The figure shows three views and two pictorial views of one solid part (mm, origin at its lowest corner). Answer the questions. A direction names the side the tool comes from. Give positions to 0.01 mm unless a question says otherwise; leave off trailing zeros. Loops run counter-clockwise (first coordinate to the right, second up) from the corner with the lowest first, then second, coordinate; pieces in that order, holes last. Notation, with made-up numbers: M 41,-40 L 63,-40 A36 ccw 63,-4 Z; hole C 46,32 d10. An arc over 180 degrees is marked long. Write item = value, one per line. Start each with the question number.
1. Section A-A on y = 20 is taken. Determine the outline of the cut face in (x, z), plus the area to 3 significant figures.
2. Section C-C on x = 194 is taken. Determine the outline of the cut face in (y, z), plus the area to 3 significant figures.
3. For the marked faces 1, 2 and 3, determine the directions among +Z, -Z, +X, -X, +Y, -Y from which every point of the face is accessible in a straight line to the end or side of a thin tool.
4. Section D-D on z = 36 is taken. Determine the outline of the cut face in (x, y).
5. Consider L1, parallel to X at y = 10, z = 30; L2, parallel to X at y = 31.5, z = 19.5; L3, parallel to Z at x = 168, y = 20. Determine where each line is inside the solid, lowest interval first. Write a range as [from, to].
6. Flat-ended cylindrical pins translate along their axes: pin 1 Ø10 at (y, z) = (4.5, 23.5) entering from +X; pin 2 Ø1.5 at (x, z) = (146.5, 31.5) entering from -Y; pin 3 Ø1 at (y, z) = (30, 31) entering from -X; pin 4 Ø4 at (x, y) = (245.5, 36) entering from -Z. Find the tip coordinate at first contact, or state that the pin passes through.
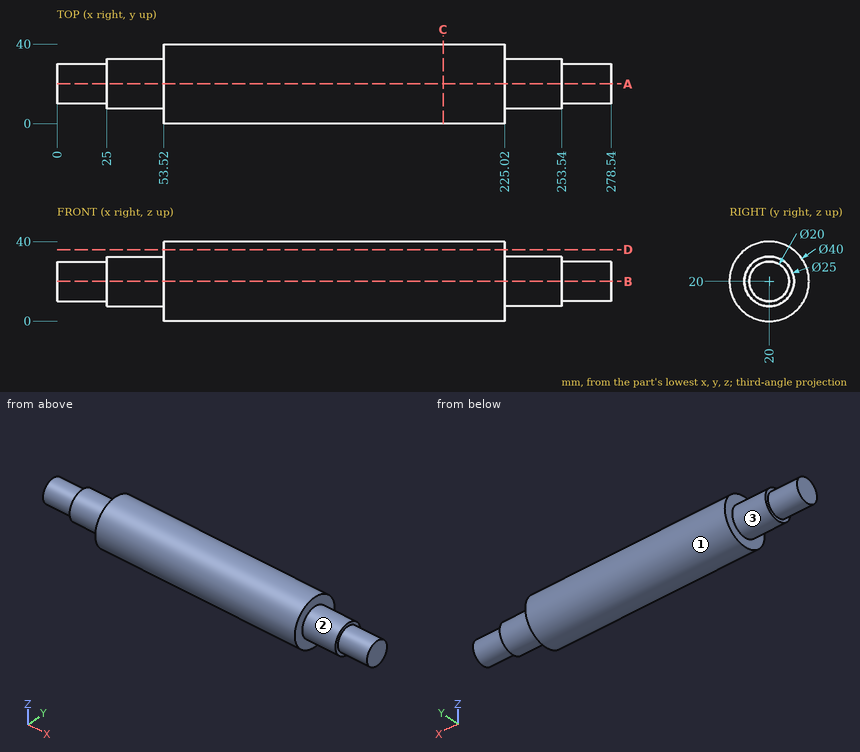
Verdict:
q1.outline = M 0,10 L 25,10 L 25,7.5 L 53.52,7.5 L 53.52,0 L 225.02,0 L 225.02,7.5 L 253.54,7.5 L 253.54,10 L 278.54,10 L 278.54,30 L 253.54,30 L 253.54,32.5 L 225.02,32.5 L 225.02,40 L 53.52,40 L 53.52,32.5 L 25,32.5 L 25,30 L 0,30 Z
q1.area = 9,290 mm2
q2.outline = C 20,20 d40
q2.area = 1,260 mm2
q3.face_1 = +X, -X
q3.face_2 = +X
q3.face_3 = -X
q4.outline = M 53.52,8 L 225.02,8 L 225.02,32 L 53.52,32 Z
q5.L1 = [53.52, 225.02]
q5.L2 = [25, 253.54]
q5.L3 = [0, 40]
q6.pin_1 = 253.54
q6.pin_2 = 3.13
q6.pin_3 = 53.52
q6.pin_4 = through
